from build123d import *

# Parameters (mm, degrees)
SKETCH1_W                                      = 60
SKETCH1_H                                      = 60
BOSS_EXTRUDE1_DEPTH                            = 3
SKETCH3_R                                      = 1
CUT_EXTRUDE3_DEPTH                             = 43.532340636
SKETCH5_R                                      = 10.25
CUT_EXTRUDE4_DEPTH                             = 43.532340636
SKETCH6_R                                      = 16
SKETCH6_R_2                                    = 10.25
BOSS_EXTRUDE2_DEPTH                            = 1
SKETCH7_R                                      = 15
SKETCH7_R_2                                    = 10.25
BOSS_EXTRUDE3_DEPTH                            = 7
SKETCH10_R                                     = 1.45
STOP_MOUNT_D2P9_THROUGH_DEPTH                  = 3.01
SKETCH11_R                                     = 2.6
STOP_MOUNT_CSK_D5P2_90DEG_DEPTH                = 1.15
STOP_MOUNT_CSK_D5P2_90DEG_DRAFT                = -45
STOP_MOUNT_CSK_D5P2_90DEG_PROFILE_2_DEPTH      = 1.15
STOP_MOUNT_CSK_D5P2_90DEG_PROFILE_2_DRAFT      = -45
SKETCH13_R                                     = 1.45
YTAB_D2P9_DEPTH                                = 3.01
SKETCH14_R                                     = 1.2
GUIDEBLOCK1_D2P4_DEPTH                         = 3.01
SKETCH15_R                                     = 2.1
GUIDEBLOCK1_HEADCOUNTERBORE_D4P2_DEPTH         = 1.5
SKETCH16_R                                     = 25.5
SKETCH16_R_2                                   = 20
ROTATING_RETAINER_HEAD_CLEARANCE_ANNULUS_DEPTH = 0.7
SKETCH17_R                                     = 1
INNER_RETAINER_M2_TAPPED_ENVELOPE_DEPTH        = 4.3
SKETCH18_R                                     = 1.46
YTAB_THROUGH_HOLE_BACKING_RESTORATION_DEPTH    = 3
SKETCH19_R                                     = 1.25
YTAB_BLIND_M2P5_THREAD_ENVELOPES_DEPTH         = 2.6


with BuildPart() as part:
    # Sketch1 → Boss-Extrude1 (new body)
    with BuildSketch(Plane(origin=(0, 0, 0), x_dir=(1, 0, 0), z_dir=(0, 1, 0))):
        Rectangle(SKETCH1_W, SKETCH1_H)
    extrude(amount=BOSS_EXTRUDE1_DEPTH)

    # Sketch3 → Cut-Extrude3 (cut, through all)
    with BuildSketch(Plane(origin=(0, 3, 0), x_dir=(1, 0, 0), z_dir=(0, 1, 0))):
        with Locations(Location((-20, 24, 0), (0, 0, 270))):
            Circle(SKETCH3_R)
        with Locations(Location((20, 24, 0), (0, 0, 270))):
            Circle(SKETCH3_R)
        with Locations(Location((-20, -24, 0), (0, 0, 270))):
            Circle(SKETCH3_R)
        with Locations(Location((20, -24, 0), (0, 0, 270))):
            Circle(SKETCH3_R)
    extrude(amount=-CUT_EXTRUDE3_DEPTH, mode=Mode.SUBTRACT)

    # Sketch5 → Cut-Extrude4 (cut, through all)
    with BuildSketch(Plane.XZ):
        with Locations(Location((0, 0, 0), (0, 0, 270))):
            Circle(SKETCH5_R)
    extrude(amount=-CUT_EXTRUDE4_DEPTH, mode=Mode.SUBTRACT)

    # Sketch6 → Boss-Extrude2 (add)
    with BuildSketch(Plane(origin=(0, 3, 0), x_dir=(1, 0, 0), z_dir=(0, 1, 0))):
        with Locations(Location((0, 0, 0), (0, 0, 270))):
            Circle(SKETCH6_R)
        with Locations(Location((0, 0, 0), (0, 0, 90))):
            Circle(SKETCH6_R_2, mode=Mode.SUBTRACT)
    extrude(amount=BOSS_EXTRUDE2_DEPTH)

    # Sketch7 → Boss-Extrude3 (add)
    with BuildSketch(Plane(origin=(0, 3, 0), x_dir=(1, 0, 0), z_dir=(0, 1, 0))):
        with Locations(Location((0, 0, 0), (0, 0, 270))):
            Circle(SKETCH7_R)
        with Locations(Location((0, 0, 0), (0, 0, 90))):
            Circle(SKETCH7_R_2, mode=Mode.SUBTRACT)
    extrude(amount=BOSS_EXTRUDE3_DEPTH)

    # Sketch10 → Stop_Mount_D2p9_Through (cut)
    with BuildSketch(Plane(origin=(0, 3, 0), x_dir=(1, 0, 0), z_dir=(0, 1, 0))):
        with Locations(Location((-24, -21, 0), (0, 0, 270))):
            Circle(SKETCH10_R)
        with Locations(Location((-27, -27, 0), (0, 0, 270))):
            Circle(SKETCH10_R)
    extrude(amount=-STOP_MOUNT_D2P9_THROUGH_DEPTH, mode=Mode.SUBTRACT)


with BuildPart() as stop_mount_csk_d5p2_90deg_tool:
    # Sketch11 → Stop_Mount_CSK_D5p2_90deg (with draft: the straight prism first)
    with BuildSketch(Plane(origin=(0, 3, 0), x_dir=(1, 0, 0), z_dir=(0, 1, 0))):
        with Locations((-24, -21)):
            Circle(SKETCH11_R)
    extrude(amount=-STOP_MOUNT_CSK_D5P2_90DEG_DEPTH)
    # Stop_Mount_CSK_D5p2_90deg: the draft: its side faces are tilted about the plane it starts from
    stop_mount_csk_d5p2_90deg_sides = [stop_mount_csk_d5p2_90deg_tool.faces().sort_by_distance(p)[0] for p in [
        (-26.6, 2.425, 21),
    ]]
    draft(stop_mount_csk_d5p2_90deg_sides, Plane(origin=(0, 3, 0), x_dir=(1, 0, 0), z_dir=(0, 1, 0)), STOP_MOUNT_CSK_D5P2_90DEG_DRAFT)


with BuildPart() as part_1:
    add(part.part)

    # Stop_Mount_CSK_D5p2_90deg: cut by stop_mount_csk_d5p2_90deg_tool
    add(stop_mount_csk_d5p2_90deg_tool.part, mode=Mode.SUBTRACT)


with BuildPart() as stop_mount_csk_d5p2_90deg_profile_2_tool:
    # Sketch11 → Stop_Mount_CSK_D5p2_90deg profile 2 (with draft: the straight prism first)
    with BuildSketch(Plane(origin=(0, 3, 0), x_dir=(1, 0, 0), z_dir=(0, 1, 0))):
        with Locations((-27, -27)):
            Circle(SKETCH11_R)
    extrude(amount=-STOP_MOUNT_CSK_D5P2_90DEG_PROFILE_2_DEPTH)
    # Stop_Mount_CSK_D5p2_90deg profile 2: the draft: its side faces are tilted about the plane it starts from
    stop_mount_csk_d5p2_90deg_profile_2_sides = [stop_mount_csk_d5p2_90deg_profile_2_tool.faces().sort_by_distance(p)[0] for p in [
        (-29.6, 2.425, 27),
    ]]
    draft(stop_mount_csk_d5p2_90deg_profile_2_sides, Plane(origin=(0, 3, 0), x_dir=(1, 0, 0), z_dir=(0, 1, 0)), STOP_MOUNT_CSK_D5P2_90DEG_PROFILE_2_DRAFT)


with BuildPart() as part_2:
    add(part_1.part)

    # Stop_Mount_CSK_D5p2_90deg profile 2: cut by stop_mount_csk_d5p2_90deg_profile_2_tool
    add(stop_mount_csk_d5p2_90deg_profile_2_tool.part, mode=Mode.SUBTRACT)

    # Sketch13 → YTab_D2p9 (cut)
    with BuildSketch(Plane.XZ):
        with Locations(Location((27, -23, 0), (0, 0, 270))):
            Circle(SKETCH13_R)
        with Locations(Location((27, -17, 0), (0, 0, 270))):
            Circle(SKETCH13_R)
    extrude(amount=-YTAB_D2P9_DEPTH, mode=Mode.SUBTRACT)

    # Sketch14 → GuideBlock1_D2p4 (cut)
    with BuildSketch(Plane(origin=(0, 3, 0), x_dir=(1, 0, 0), z_dir=(0, 1, 0))):
        with Locations(Location((28, 0, 0), (0, 0, 270))):
            Circle(SKETCH14_R)
        with Locations(Location((20, 0, 0), (0, 0, 270))):
            Circle(SKETCH14_R)
    extrude(amount=-GUIDEBLOCK1_D2P4_DEPTH, mode=Mode.SUBTRACT)

    # Sketch15 → GuideBlock1_HeadCounterbore_D4p2 (cut)
    with BuildSketch(Plane(origin=(0, 3, 0), x_dir=(1, 0, 0), z_dir=(0, 1, 0))):
        with Locations((28, 0)):
            Circle(SKETCH15_R)
        with Locations(Location((20, 0, 0), (0, 0, 270))):
            Circle(SKETCH15_R)
    extrude(amount=-GUIDEBLOCK1_HEADCOUNTERBORE_D4P2_DEPTH, mode=Mode.SUBTRACT)

    # Sketch16 → Rotating_Retainer_Head_Clearance_Annulus (cut)
    with BuildSketch(Plane(origin=(0, 3, 0), x_dir=(1, 0, 0), z_dir=(0, 1, 0))):
        with Locations(Location((0, 0, 0), (0, 0, 270))):
            Circle(SKETCH16_R)
        Circle(SKETCH16_R_2, mode=Mode.SUBTRACT)
    extrude(amount=-ROTATING_RETAINER_HEAD_CLEARANCE_ANNULUS_DEPTH, mode=Mode.SUBTRACT)

    # Sketch17 → Inner_Retainer_M2_Tapped_Envelope (cut)
    with BuildSketch(Plane(origin=(0, 10, 0), x_dir=(1, 0, 0), z_dir=(0, 1, 0))):
        with Locations(Location((-9.399263552, -8.240378916, 0), (0, 0, 270))):
            Circle(SKETCH17_R)
        with Locations(Location((-2.436745703, 12.260190471, 0), (0, 0, 270))):
            Circle(SKETCH17_R)
        with Locations(Location((11.836009254, -4.019811554, 0), (0, 0, 270))):
            Circle(SKETCH17_R)
    extrude(amount=-INNER_RETAINER_M2_TAPPED_ENVELOPE_DEPTH, mode=Mode.SUBTRACT)

    # Sketch18 → YTab_Through_Hole_Backing_Restoration (add)
    with BuildSketch(Plane.XZ):
        with Locations((27, -23)):
            Circle(SKETCH18_R)
        with Locations((27, -17)):
            Circle(SKETCH18_R)
    extrude(amount=-YTAB_THROUGH_HOLE_BACKING_RESTORATION_DEPTH)

    # Sketch19 → YTab_Blind_M2p5_Thread_Envelopes (cut)
    with BuildSketch(Plane.XZ):
        with Locations(Location((27, -23, 0), (0, 0, 270))):
            Circle(SKETCH19_R)
        with Locations(Location((27, -17, 0), (0, 0, 270))):
            Circle(SKETCH19_R)
    extrude(amount=-YTAB_BLIND_M2P5_THREAD_ENVELOPES_DEPTH, mode=Mode.SUBTRACT)


solid = part_2.part
Can you work these out from the model? Positions are in its coordinate system, mm. A direction names the side the tool comes from. Round coordinates to 2 decimals unless told otherwise and drop trailing zeros. Loops run counter-clockwise (first coordinate to the right, second up) from the corner with the lowest first, then second, coordinate; pieces in that order, holes last. Notation, with made-up numbers: (-32, -14) - (23, -14) arc R20 cw to (23, 23) - close; hole circle Ø5 at (61, 69.25). An arc over 180 degrees is marked (long way). Answer in a Markdown table with one row per item. Add a question column.
Q1. I want a section at C-C on y = 7.25. List the corners of the cut face in (x, z) for me.
Q2. We'd pull the mould along Z, two halves only. Please class faces 1 (the flat face through (-6, 3, -15)), 2 (the cylindrical face through (12.827, 7.88, 3.89)), 3 (the cylindrical face through (0.66, 6.958, -14.985)): pulls with the +Z half, pulls with the -Z half, needs draft (parallel to the pull), parting line crosses it, or undercut.
Q3. For pin 1 Ø6 at (x, y) = (-3, 9) entering from +Z; pin 2 Ø4 at (x, z) = (20, 0) entering from +Y; pin 3 Ø4 at (x, y) = (11, 7) entering from -Z, each with a flat end and sliding along its axis, tell me the tip position at first contact or that it passes through.
Q4. Which directions (+Z, -Z, +X, -X, +Y, -Y) give clear straight access to the entire face, cutting with the end or side of a thin tool? Please do faces 4 (the flat face through (27, 2.6, -23)), 5 (the cylindrical face through (-24.9, 2.7, -5.5)), 6 (the cylindrical face through (26.935, 0.76, 0.554)).
Q5. I want a section at D-D on z = 27. List the corners of the cut face in (x, y) for me.
Q6. I want a section at A-A on x = 0. List the corners of the cut face in (y, z) for me.
Q7. I need wall thicknesses on L1, parallel to X at y = 0.4, z = 0; L2, parallel to X at y = 1.85, z = 24; L3, parallel to X at y = 2.15, z = 0. Which ranges of each line are inside material? Lowest first, please.
Q8. I want a section at B-B on z = -5. List the corners of the cut face in (x, y) for me (3 decimals).
A:
| question | item | result |
|---|---|---|
| 1 | outline | circle Ø30 at (0, 0); hole circle Ø2 at (-9.4, 8.24); hole circle Ø20.5 at (0, 0); hole circle Ø2 at (-2.44, -12.26); hole circle Ø2 at (11.84, 4.02) |
| 2 | face 1 | needs draft |
| 2 | face 2 | undercut |
| 2 | face 3 | parting line crosses it |
| 3 | pin 1 | z = 15 |
| 3 | pin 2 | y = 1.5 |
| 3 | pin 3 | z = -12 |
| 4 | face 4 | -Y |
| 4 | face 5 | +Y |
| 4 | face 6 | +Y, -Y |
| 5 | outline | (-30, 0) - (-28.45, 0) - (-28.45, 1.85) - (-29.6, 3) - (-30, 3) - close; (-25.55, 0) - (30, 0) - (30, 3) - (-24.4, 3) - (-25.55, 1.85) - close |
| 6 | outline | (0, -30) - (3, -30) - (3, -25.5) - (2.3, -25.5) - (2.3, -20) - (3, -20) - (3, -16) - (4, -16) - (4, -15) - (10, -15) - (10, -10.25) - (0, -10.25) - close; (0, 10.25) - (10, 10.25) - (10, 15) - (4, 15) - (4, 16) - (3, 16) - (3, 20) - (2.3, 20) - (2.3, 25.5) - (3, 25.5) - (3, 30) - (0, 30) - close |
| 7 | L1 | -30 to -10.25, 10.25 to 18.8, 21.2 to 26.8, 29.2 to 30 |
| 7 | L2 | -30 to -21, -19 to 19, 21 to 30 |
| 7 | L3 | -30 to -10.25, 10.25 to 17.9, 22.1 to 25.9 |
| 8 | outline | (-30, 0) - (-8.948, 0) - (-8.948, 10) - (-14.142, 10) - (-14.142, 4) - (-15.199, 4) - (-15.199, 3) - (-19.365, 3) - (-19.365, 2.3) - (-25.005, 2.3) - (-25.005, 3) - (-30, 3) - close; (8.948, 0) - (30, 0) - (30, 3) - (25.005, 3) - (25.005, 2.3) - (19.365, 2.3) - (19.365, 3) - (15.199, 3) - (15.199, 4) - (14.142, 4) - (14.142, 10) - (8.948, 10) - close |
